```python
from build123d import *

# Parameters (mm, degrees)
ESBO_O1_W                         = 30
ESBO_O1_H                         = 30
RESSALTO_EXTRUS_O1_DEPTH          = 50
ESBO_O2_W                         = 25
ESBO_O2_H                         = 5
CORTE_EXTRUS_O1_DEPTH             = 31
ESBO_O3_W                         = 25
ESBO_O3_H                         = 25
CORTE_EXTRUS_O2_DEPTH             = 25
FURO_COM_FOLGA_DE_M41_D           = 4.5
FURO_COM_FOLGA_DE_M41_ON_FACE_2_D = 4.5


with BuildPart() as part:
    # Esboço1 → Ressalto-extrusão1 (new body)
    with BuildSketch(Plane.XY):
        with Locations((-15, 15)):
            Rectangle(ESBO_O1_W, ESBO_O1_H)
    extrude(amount=RESSALTO_EXTRUS_O1_DEPTH)

    # Esboço2 → Corte-extrusão1 (cut, through all)
    with BuildSketch(Plane(origin=(0, 30, 0), x_dir=(1, 0, 0), z_dir=(0, 1, 0))):
        with Locations((-17.5, -12.5)):
            Rectangle(ESBO_O2_W, ESBO_O2_H)
    extrude(amount=-CORTE_EXTRUS_O1_DEPTH, mode=Mode.SUBTRACT)

    # Esboço3 → Corte-extrusão2 (cut)
    with BuildSketch(Plane(origin=(0, 30, 0), x_dir=(1, 0, 0), z_dir=(0, 1, 0))):
        with Locations((-17.5, -37.5)):
            Rectangle(ESBO_O3_W, ESBO_O3_H)
    extrude(amount=-CORTE_EXTRUS_O2_DEPTH, mode=Mode.SUBTRACT)

    # Furo com folga de M41 (through all)
    with Locations(Plane(origin=(-15, 5, 35), x_dir=(0, 0, 1), z_dir=(0, 1, 0))):
        with Locations((0, 0)):
            Hole(FURO_COM_FOLGA_DE_M41_D / 2)

    # Furo com folga de M41 on face 2 (through all)
    with Locations(Plane(origin=(-5, 15, 35), x_dir=(0, 0, -1), z_dir=(-1, 0, 0))):
        with Locations((0, 0)):
            Hole(FURO_COM_FOLGA_DE_M41_ON_FACE_2_D / 2)


solid = part.part
```
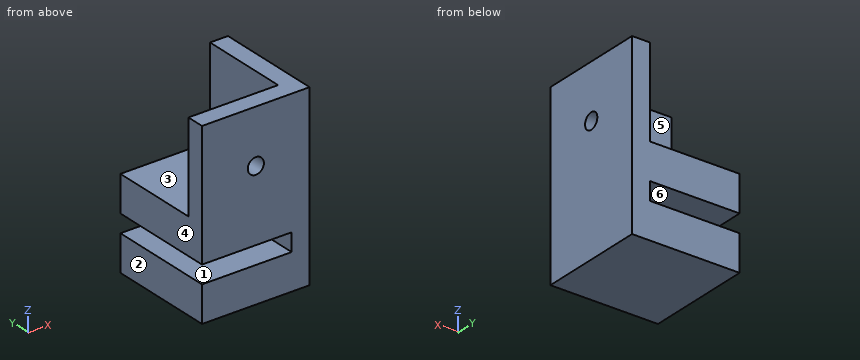
Check sheet for the modelled part. Datum: model origin and axes. Units: mm. Face numbers are marked on the shaded views. A direction names the side the tool comes from. Give positions to 0.01 mm unless a question says otherwise; leave off trailing zeros. Write each loop counter-clockwise with the first axis right and the second up, starting at its lowest first coordinate (ties: lowest second). Pieces come first, ordered by that corner, then holes. Notation, with made-up numbers: (-21.75, 3.25) - (8.25, 3.25) arc R18 ccw to (8.25, 26.25) - close; hole circle Ø10 at (59.25, -3.5). An arc over 180 degrees is marked (long way). Answer as a JSON object with one key per item and string values. Group by question number.
1) Sectioned sample at D-D (x = -28). Record the cut outline in (y, z), then the cut area to 3 significant figures.
2) Access from +Z, -Z, +X, -X, +Y, -Y to the whole of each face (thin tool, end or side, straight path). Record for the marked faces 4, 5 and 6.
3) Sectioned sample at A-A (z = 35). Record the cut outline in (x, y), then the cut area to 3 significant figures.
4) Release check for a two-part mould opening along Z. For the marked faces 1, 2 and 3 record: pulls with the +Z half, pulls with the -Z half, needs draft (parallel to the pull), parting line crosses it, or undercut.
5) Depth check by flat-ended pin: P1, Ø4, axis at y = 9, z = 12.5, coming from the -X side; P2, Ø12.5, axis at x = -21, y = 17, coming from the +Z side; P3, Ø2, axis at x = -7.5, z = 37, coming from the +Y side. Enter the tip coordinate at first touch or a pass-through.
6) Sectioned sample at B-B (x = -15). Record the cut outline in (y, z).
7) Thickness scan on probe 1 along X at (y, z) = (2.75, 35); probe 2 along Y at (x, z) = (-2.2, 35); probe 3 along Z at (x, y) = (-9.5, 10.5). Record the ranges inside material, lowest first. Write a range as from..to.
8) Sectioned sample at C-C (y = 15). Record the cut outline in (x, z), then the cut area to 4 significant figures.
Geometry results:
{
 "1": {"outline": "(0, 0) - (30, 0) - (30, 10) - (0, 10) - close; (0, 15) - (30, 15) - (30, 25) - (5, 25) - (5, 50) - (0, 50) - close", "area": "725 mm^2"},
 "2": {"face 4": "+Z, -Z, -X, +Y, -Y", "face 5": "+Z, -X, +Y", "face 6": "-X, +Y, -Y"},
 "3": {"outline": "(-30, 0) - (-17.25, 0) - (-17.25, 5) - (-30, 5) - close; (-12.75, 0) - (0, 0) - (0, 12.75) - (-5, 12.75) - (-5, 5) - (-12.75, 5) - close; (-5, 17.25) - (0, 17.25) - (0, 30) - (-5, 30) - close", "area": "230 mm^2"},
 "4": {"face 1": "undercut", "face 2": "needs draft", "face 3": "pulls with the +Z half"},
 "5": {"P1": "stops at x = -5", "P2": "stops at z = 25", "P3": "stops at y = 5"},
 "6": {"outline": "(0, 0) - (30, 0) - (30, 10) - (0, 10) - close; (0, 15) - (30, 15) - (30, 25) - (5, 25) - (5, 32.75) - (0, 32.75) - close; (0, 37.25) - (5, 37.25) - (5, 50) - (0, 50) - close"},
 "7": {"probe 1": "x = -30..-17.25, -12.75..0", "probe 2": "y = 0..12.75, 17.25..30", "probe 3": "z = 0..10, 15..25"},
 "8": {"outline": "(-30, 0) - (0, 0) - (0, 32.75) - (-5, 32.75) - (-5, 25) - (-30, 25) - (-30, 15) - (-5, 15) - (-5, 10) - (-30, 10) - close; (-5, 37.25) - (0, 37.25) - (0, 50) - (-5, 50) - close", "area": "727.5 mm^2"}
}
